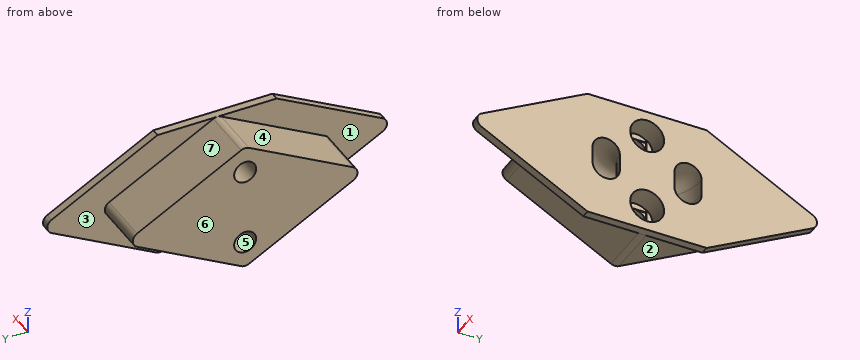
```python
from build123d import *
from build123d.topology import SkipClean

# Parameters (mm, degrees)
BOSS_EXTRUDE1_DEPTH = 12.446
BOSS_EXTRUDE3_DEPTH = 1.905
FILLET1_R           = 1.905
SKETCH8_R           = 3.937
CUT_EXTRUDE3_DEPTH  = 5.08
SKETCH9_R           = 2.5527
CUT_EXTRUDE4_DEPTH  = 47.270145624
CUT_EXTRUDE7_DEPTH  = 48.009337913
CUT_EXTRUDE8_DEPTH  = 0.2
SKETCH14_W          = 5.1054
SKETCH14_H          = 5.1054
CUT_EXTRUDE9_DEPTH  = 0.2


with BuildPart() as part:
    # Sketch1 → Boss-Extrude1 (new body)
    with BuildSketch(Plane(origin=(0, 0, 0), x_dir=(0, 0, -1), z_dir=(1, 0, 0))):
        Polygon((0, -28.2575), (15.24, 0), (0, 28.2575), (-15.24, 0), align=None)
    extrude(amount=BOSS_EXTRUDE1_DEPTH)

    # Sketch6 → Boss-Extrude3 (add)
    with BuildSketch(Plane(origin=(12.446, 0, 0), x_dir=(0, 0, -1), z_dir=(1, 0, 0))):
        Polygon((-22.454651823, 0), (0, -41.634666921), (22.454651823, 0), (0, 41.634666921), align=None)
    extrude(amount=BOSS_EXTRUDE3_DEPTH)

    # Fillet1
    fillet1_edges = [part.edges().sort_by_distance(p)[0] for p in [
        (13.3985, 41.634666921, 0),
        (13.3985, 0, 22.454651823),
        (13.3985, -41.634666921, 0),
        (13.3985, 0, -22.454651823),
        (6.223, 0, -15.24),
        (6.223, -28.2575, 0),
        (6.223, 0, 15.24),
        (6.223, 28.2575, 0),
    ]]
    fillet(fillet1_edges, radius=FILLET1_R)

    # Sketch7 → Cut-Revolve2 (revolve, cut)
    with BuildSketch(Plane(origin=(0, 0, 0), x_dir=(1, 0, 0), z_dir=(0, 1, 0))):
        with BuildLine():
            Line((1.651, -1.905), (1.651, 1.905))
            ThreePointArc((1.651, 1.905), (4.826, 5.08), (8.001, 1.905))
            Line((8.001, 1.905), (8.001, -1.905))
            ThreePointArc((8.001, -1.905), (4.826, -5.08), (1.651, -1.905))
        make_face()
    revolve(axis=Axis((14.351, 0, 0), (0, 0, 1)), mode=Mode.SUBTRACT)

    # Sketch8 → Cut-Extrude3 (cut)
    with BuildSketch(Plane(origin=(14.351, 0, 0), x_dir=(0, 0, -1), z_dir=(1, 0, 0))):
        with Locations((8.89, 0)):
            Circle(SKETCH8_R)
        with Locations(Location((-8.89, 0, 0), (0, 0, 180))):
            Circle(SKETCH8_R)
    extrude(amount=-CUT_EXTRUDE3_DEPTH, mode=Mode.SUBTRACT)

    # Sketch9 → Cut-Extrude4 (cut, through all)
    with BuildSketch(Plane(origin=(9.271, 0, 0), x_dir=(0, 0, -1), z_dir=(1, 0, 0))):
        with Locations((8.89, 0)):
            Circle(SKETCH9_R)
        with Locations(Location((-8.89, 0, 0), (0, 0, 180))):
            Circle(SKETCH9_R)
    extrude(amount=-CUT_EXTRUDE4_DEPTH, mode=Mode.SUBTRACT)

    # Sketch12 → Cut-Extrude7 (cut, through all)
    with BuildSketch(Plane.ZY.offset(-12.446)):
        with BuildLine():
            Line((-14.980604453, -13.858129497), (-14.980604453, 13.858129497))
            Line((-14.980604453, 13.858129497), (-21.966948415, 0.904283401))
            ThreePointArc((-21.966948415, 0.904283401), (-22.195256276, 0), (-21.966948415, -0.904283401))
            Line((-21.966948415, -0.904283401), (-14.980604453, -13.858129497))
        make_face()
        with BuildLine():
            Line((14.980604453, -13.858129497), (14.980604453, 13.858129497))
            Line((14.980604453, 13.858129497), (21.966948415, 0.904283401))
            ThreePointArc((21.966948415, 0.904283401), (22.195256276, 0), (21.966948415, -0.904283401))
            Line((21.966948415, -0.904283401), (14.980604453, -13.858129497))
        make_face()
    extrude(amount=-CUT_EXTRUDE7_DEPTH, mode=Mode.SUBTRACT)

    # Sketch13 → Cut-Extrude8 (cut)
    with SkipClean():  # the faces are left unmerged after this step: merging them gives an invalid solid
        with BuildSketch(Plane(origin=(9.271, 0, 0), x_dir=(0, 0, -1), z_dir=(1, 0, 0))):
            with BuildLine():
                Line((5.892719281, 2.5527), (11.887280719, 2.5527))
                ThreePointArc((11.887280719, 2.5527), (12.827, 0), (11.887280719, -2.5527))
                Line((11.887280719, -2.5527), (5.892719281, -2.5527))
                ThreePointArc((5.892719281, -2.5527), (4.953, 0), (5.892719281, 2.5527))
            make_face()
            with BuildLine():
                Line((-11.887280719, 2.5527), (-5.892719281, 2.5527))
                ThreePointArc((-5.892719281, 2.5527), (-4.953, 0), (-5.892719281, -2.5527))
                Line((-5.892719281, -2.5527), (-11.887280719, -2.5527))
                ThreePointArc((-11.887280719, -2.5527), (-12.827, 0), (-11.887280719, 2.5527))
            make_face()
        extrude(amount=-CUT_EXTRUDE8_DEPTH, mode=Mode.SUBTRACT)

    # Sketch14 → Cut-Extrude9 (cut)
    with SkipClean():  # the faces are left unmerged after this step: merging them gives an invalid solid
        with BuildSketch(Plane(origin=(9.071, 0, 0), x_dir=(0, 0, -1), z_dir=(1, 0, 0))):
            with Locations((8.89, 0)):
                Rectangle(SKETCH14_W, SKETCH14_H)
            with Locations((-8.89, 0)):
                Rectangle(SKETCH14_W, SKETCH14_H)
        extrude(amount=-CUT_EXTRUDE9_DEPTH, mode=Mode.SUBTRACT)


solid = part.part
```
Can you work these out from the model? Positions are in its coordinate system, mm. Face numbers are marked on the shaded views. A direction names the side the tool comes from. Coordinates: 2 decimals unless noted, no trailing zeros. Order: outer loops, then holes, each group sorted by start corner. A loop starts at its lowest first (then second) coordinate and runs counter-clockwise, first axis right, second up. Notation, with made-up numbers: (60.5, 84.5) -> (87.5, 84.5) arc R21 ccw to (87.5, 104.5) -> close; hole circle Ø6 at (-33, 83.25). An arc over 180 degrees is marked (long way). Write each question's results on one line, items separated by ' | '.
Item 1: Which directions (+Z, -Z, +X, -X, +Y, -Y) give clear straight access to the entire face, cutting with the end or side of a thin tool? Please do the marked faces 1, 2, 3 and 4.
Results are:
face 1: -X, -Y | face 2: -Z, -X, +Y | face 3: -X, +Y | face 4: +Z, -X, -Y
Item 2: I want a section at C-C, the plane y = 32. Write out the boundary of the cut face in (x, z).
Results are:
outline: (12.45, -5.2) -> (14.35, -5.2) -> (14.35, 5.2) -> (12.45, 5.2) -> close
Item 3: If we mould it in two halves opening along Z, with no side actions, what happens to the marked faces 5, 6 and 7? For each: +Z half, -Z half, draft (parallel to the pull), parting line (faces both ways), or undercut.
Results are:
face 5: undercut | face 6: draft | face 7: +Z half
Item 4: I want a section at B-B, the plane z = 3.25. Write out the boundary of the cut face in (x, y), then the cut area to 3 significant figures.
Results are:
outline: (0, -22.23) -> (12.45, -22.23) -> (12.45, -35.61) -> (14.35, -35.61) -> (14.35, -12.4) arc R12.4 cw to (14.35, 12.4) -> (14.35, 35.61) -> (12.45, 35.61) -> (12.45, 22.23) -> (0, 22.23) -> close; (14.35, -6.65) -> (14.35, 6.65) arc R6.65 ccw to start | area: 517 mm²
Item 5: I'm going to push flat-ended pins straight in: pin 1 Ø2 at (x, z) = (11, -11.5) entering from -Y; pin 2 Ø0.7 at (y, z) = (-0.5, -5.5) entering from +X; pin 3 Ø0.8 at (y, z) = (1, 10.5) entering from +X; pin 4 Ø3 at (x, y) = (3, -4.5) entering from -Z. Where does each tip first touch, or does it pass through?
Results are:
pin 1: y = -8.79 | pin 2: x = 9.07 | pin 3: through | pin 4: z = -13.62
Item 6: I want a section at D-D, the plane x = 10.25. Count the separate pieces of the cut face and the enclosed holes in it, then the cut area to 3 significant figures.
Results are:
separate pieces: 1 | enclosed holes: 4 | area: 632 mm²
Item 7: I want a section at A-A, the plane z = -10.75. Write out the boundary of the cut face in (x, y).
Results are:
outline: (0, -8.33) -> (12.45, -8.33) -> (12.45, -21.7) -> (14.35, -21.7) -> (14.35, -3.47) -> (9.27, -3.47) -> (9.27, -2.55) -> (8.87, -2.55) -> (8.87, -1.75) -> (0, -1.75) -> close; (0, 1.75) -> (8.87, 1.75) -> (8.87, 2.55) -> (9.27, 2.55) -> (9.27, 3.47) -> (14.35, 3.47) -> (14.35, 21.7) -> (12.45, 21.7) -> (12.45, 8.33) -> (0, 8.33) -> close
Item 8: If I drill on line 1 along Z through (x, y) = (6.5, 2); line 2 along Z through (x, y) = (5, 1); line 3 along X through (y, z) = (-12, -9.5), over which ranges is the centre line in solid material (lowest first)?
Results are:
line 1: -14.16 to -10.48, -7.3 to -4.74, 4.74 to 7.3, 10.48 to 14.16 | line 2: -14.7 to -11.24, -6.54 to -5.08, 5.08 to 6.54, 11.24 to 14.7 | line 3: 12.45 to 14.35
